CAD build for the part. Positions are in the model's coordinates, mm. Give positions to 0.01 mm unless a question says otherwise; leave off trailing zeros. Order: outer loops, then holes, each group sorted by start corner. A loop starts at its lowest first (then second) coordinate and runs counter-clockwise, first axis right, second up.
from build123d import *

# Parameters (mm, degrees)
F0_W     = 62.156647
F0_H     = 31.778897
F0_R     = 5.974125
F0_R_2   = 8.570031
F0_R_3   = 5.457517
F1_DEPTH = 6.35
F2_DEPTH = 25.4


with BuildPart() as f1:
    # F0 (on Top) → F1 (new body)
    with BuildSketch(Plane.XY):
        with Locations((-56.918233, -40.388333)):
            Rectangle(F0_W, F0_H)
        with Locations((-35.330459, -49.565207)):
            Circle(F0_R, mode=Mode.SUBTRACT)
        with Locations((-72.268285, -40.162876)):
            Circle(F0_R_2, mode=Mode.SUBTRACT)
        with Locations((-34.6459, -31.120101)):
            Circle(F0_R_3, mode=Mode.SUBTRACT)
    extrude(amount=F1_DEPTH)

    # F0 (on Top) → F2 (join)
    with BuildSketch(Plane.XY):
        with Locations((-56.918233, -40.388333)):
            Rectangle(F0_W, F0_H)
        with Locations((-35.330459, -49.565207)):
            Circle(F0_R, mode=Mode.SUBTRACT)
        with Locations((-72.268285, -40.162876)):
            Circle(F0_R_2, mode=Mode.SUBTRACT)
        with Locations((-34.6459, -31.120101)):
            Circle(F0_R_3, mode=Mode.SUBTRACT)
    extrude(amount=F2_DEPTH)


solid = f1.part
1. Saw through at C-C on x = -73. Give the cut face in (y, z), plus the area to 3 significant figures.
2. Saw through at A-A on y = -38.5. Give the cut face in (x, z), plus the area to 3 significant figures.
3. Wall check: line 1 (X direction, y = -31.5, z = 21.5); line 2 (Y direction, x = -30, z = 9.25); line 3 (X direction, y = -32.5, z = 18.25). Give the ranges that are in metal, low to high.
4. Saw through at D-D on z = 20.75. Give the cut face in (x, y), plus the area to 3 significant figures.
5. Mould opens along Y. For faces 1 (the flat face through (-57, -40, 0)), 2 (the flat face through (-57, -56.278, 13)), 3 (the cylindrical face through (-74.13, -48.53, 12.52)) say: released by +Y, released by -Y, zero draft, split by the parting line, or undercut.
6. Pin check, flat tip, straight feed: P1, Ø13.5, axis at x = -72.27, y = -40.16, coming from the +Z side. Stop position of the tip, or through.
7. Saw through at B-B on y = -46. Give the cut face in (x, z), plus the area to 3 significant figures.
Reported:
1. outline: (-56.28, 0) - (-48.7, 0) - (-48.7, 25.4) - (-56.28, 25.4) - close; (-31.62, 0) - (-24.5, 0) - (-24.5, 25.4) - (-31.62, 25.4) - close
1. area: 373 mm2
2. outline: (-88, 0) - (-80.68, 0) - (-80.68, 25.4) - (-88, 25.4) - close; (-63.86, 0) - (-25.84, 0) - (-25.84, 25.4) - (-63.86, 25.4) - close
2. area: 1,150 mm2
3. line 1: x = -88 to -40.09, -29.2 to -25.84
3. line 2: y = -56.28 to -52.26, -46.87 to -33.98, -28.26 to -24.5
3. line 3: x = -88 to -76.11, -68.43 to -39.93, -29.37 to -25.84
4. outline: (-88, -56.28) - (-25.84, -56.28) - (-25.84, -24.5) - (-88, -24.5) - close; hole circle Ø17.14 at (-72.27, -40.16); hole circle Ø11.95 at (-35.33, -49.57); hole circle Ø10.92 at (-34.65, -31.12)
4. area: 1,540 mm2
5. face 1: zero draft
5. face 2: released by -Y
5. face 3: undercut
6. P1: passes through
7. outline: (-88, 0) - (-78.54, 0) - (-78.54, 25.4) - (-88, 25.4) - close; (-65.99, 0) - (-40.12, 0) - (-40.12, 25.4) - (-65.99, 25.4) - close; (-30.54, 0) - (-25.84, 0) - (-25.84, 25.4) - (-30.54, 25.4) - close
7. area: 1,020 mm2
